The listing builds one solid part. Answer for the finished solid, in the listing's coordinates (mm). A direction names the side the tool comes from. Give positions to 0.01 mm unless a question says otherwise; leave off trailing zeros. Order: outer loops, then holes, each group sorted by start corner. A loop starts at its lowest first (then second) coordinate and runs counter-clockwise, first axis right, second up. Notation, with made-up numbers: (61.25, 46) - (76.25, 46) arc R16 cw to (76.25, 59) - close; hole circle Ø2 at (32.25, 13.25). An arc over 180 degrees is marked (long way). Answer as a JSON object with one key per item and string values. Group by question number.
Q1. The mould has two halves that part along X. Classify faces 4 (the face through (-0.1, 12.3, 1.5)), 5 (the face through (-2.38, -10.74, -2.46)), 6 (the face through (-15, 0, 1)): released by +X, released by -X, zero draft, split by the parting line, or undercut.
Q2. Given pin 1 (4 mm diameter, centred on x = -10.5, y = -10.5, fed in from -Z); pin 2 (5 mm diameter, centred on x = -5.5, z = -5, fed in from -Y); pin 3 (5 mm diameter, centred on x = -2.5, z = -4.5, fed in from +Y); pin 4 (1 mm diameter, centred on x = -10.5, y = -9.5, fed in from -Z), each flat-ended and moving along its own axis, determine where each tip first touches the part or whether it passes through.
Q3. Consider line 1 (Y direction, x = 0, z = -2.1); line 2 (Z direction, x = -1, y = 8.5); line 3 (Z direction, x = -6.5, y = 13). Determine where each line is inside the solid, lowest interval first.
Q4. A cutting plane is placed at B-B, the plane x = -9.5. Count the separate pieces of the cut face and the enclosed holes in it, and give its area (3 significant figures).
Q5. A cutting plane is placed at A-A, the plane z = -1.5. Give the vertices of the cut face in (x, y), and give its area (3 significant figures).
Q6. For faces 1 (the face through (12.4, -12.43, 0.74)), 2 (the face through (0, 11.5, -4)), 3 (the face through (1, 12, 0)), determine the directions among +Z, -Z, +X, -X, +Y, -Y from which every point of the face is accessible in a straight line to the end or side of a thin tool.
from build123d import *

# Parameters (mm, degrees)
ESQUISSE1_R             = 1.75
BASE_EXTRUSION_DEPTH    = 1.5
ESQUISSE2_R             = 12.5
BOSS_EXTRU_1_DEPTH      = 8
CHANFREIN1_SIZE         = 1
ESQUISSE3_R             = 11
ENL_V_MAT_EXTRU_1_DEPTH = 8
CONG_1_R                = 1
ESQUISSE4_W             = 15.143469624
ESQUISSE4_H             = 5.581450233
ENL_V_MAT_EXTRU_3_DEPTH = 8


with BuildPart() as part:
    # Esquisse1 → Base-Extrusion (new body)
    with BuildSketch(Plane.XY):
        with BuildLine():
            Line((-11.405090569, -12.958545795), (-3.038179265, -14.689093463))
            ThreePointArc((-3.038179265, -14.689093463), (0, -15), (3.038179265, -14.689093463))
            Line((3.038179265, -14.689093463), (11.405090569, -12.958545795))
            ThreePointArc((11.405090569, -12.958545795), (12.414213562, -12.414213562), (12.958545795, -11.405090569))
            Line((12.958545795, -11.405090569), (14.689093463, -3.038179265))
            ThreePointArc((14.689093463, -3.038179265), (15, 0), (14.689093463, 3.038179265))
            Line((14.689093463, 3.038179265), (12.958545795, 11.405090569))
            ThreePointArc((12.958545795, 11.405090569), (12.414213562, 12.414213562), (11.405090569, 12.958545795))
            Line((11.405090569, 12.958545795), (3.038179265, 14.689093463))
            ThreePointArc((3.038179265, 14.689093463), (0, 15), (-3.038179265, 14.689093463))
            Line((-3.038179265, 14.689093463), (-11.405090569, 12.958545795))
            ThreePointArc((-11.405090569, 12.958545795), (-12.414213562, 12.414213562), (-12.958545795, 11.405090569))
            Line((-12.958545795, 11.405090569), (-14.689093463, 3.038179265))
            ThreePointArc((-14.689093463, 3.038179265), (-15, 0), (-14.689093463, -3.038179265))
            Line((-14.689093463, -3.038179265), (-12.958545795, -11.405090569))
            ThreePointArc((-12.958545795, -11.405090569), (-12.414213562, -12.414213562), (-11.405090569, -12.958545795))
        make_face()
        with Locations((-10.5, 10.5)):
            Circle(ESQUISSE1_R, mode=Mode.SUBTRACT)
        with Locations((10.5, 10.5)):
            Circle(ESQUISSE1_R, mode=Mode.SUBTRACT)
        with Locations((-10.5, -10.5)):
            Circle(ESQUISSE1_R, mode=Mode.SUBTRACT)
        with Locations((10.5, -10.5)):
            Circle(ESQUISSE1_R, mode=Mode.SUBTRACT)
    extrude(amount=BASE_EXTRUSION_DEPTH)

    # Esquisse2 → Boss.-Extru.1 (add)
    with BuildSketch(Plane(origin=(0, 0, 0), x_dir=(-1, 0, 0), z_dir=(0, 0, -1))):
        with Locations(Location((0, 0, 0), (0, 0, 180))):
            Circle(ESQUISSE2_R)
    extrude(amount=BOSS_EXTRU_1_DEPTH)

    # Chanfrein1
    chanfrein1_edges = [part.edges().sort_by_distance(p)[0] for p in [
        (-12.5, 0, -8),
    ]]
    chamfer(chanfrein1_edges, length=CHANFREIN1_SIZE)

    # Esquisse3 → Enlèv. mat.-Extru.1 (cut)
    with BuildSketch(Plane.XY.offset(1.5)):
        Circle(ESQUISSE3_R)
    extrude(amount=-ENL_V_MAT_EXTRU_1_DEPTH, mode=Mode.SUBTRACT)

    # Congé1
    cong_1_edges = [part.edges().sort_by_distance(p)[0] for p in [
        (-11, 0, -6.5),
        (-11, 0, 1.5),
    ]]
    fillet(cong_1_edges, radius=CONG_1_R)

    # Esquisse4 → Enlèv. mat.-Extru.3 (cut)
    with BuildSketch(Plane(origin=(0, 0, 0), x_dir=(-1, 0, 0), z_dir=(0, 0, -1))):
        with Locations((-0.10816764, 14.290725117)):
            Rectangle(ESQUISSE4_W, ESQUISSE4_H)
    extrude(amount=ENL_V_MAT_EXTRU_3_DEPTH, mode=Mode.SUBTRACT)


solid = part.part
Reply:
{
 "1": {"face 4": "zero draft", "face 5": "undercut", "face 6": "released by -X"},
 "2": {"pin 1": "stops at z = 0", "pin 2": "stops at y = -12.13", "pin 3": "stops at y = 11.5", "pin 4": "passes through"},
 "3": {"line 1": "y = -12.5 to -11, 11 to 11.5", "line 2": "z = -8 to -6.5", "line 3": "z = 0 to 1.5"},
 "4": {"separate pieces": "3", "enclosed holes": "0", "area": "71.2 mm^2"},
 "5": {"outline": "(-4.9, 11.5) arc R12.5 ccw (long way) to (4.9, 11.5) - close; hole circle Ø22 at (0, 0)", "area": "104 mm^2"},
 "6": {"face 1": "+Z, -Z, +X, -Y", "face 2": "-Z, +X, -X, +Y", "face 3": "-Z"}
}
